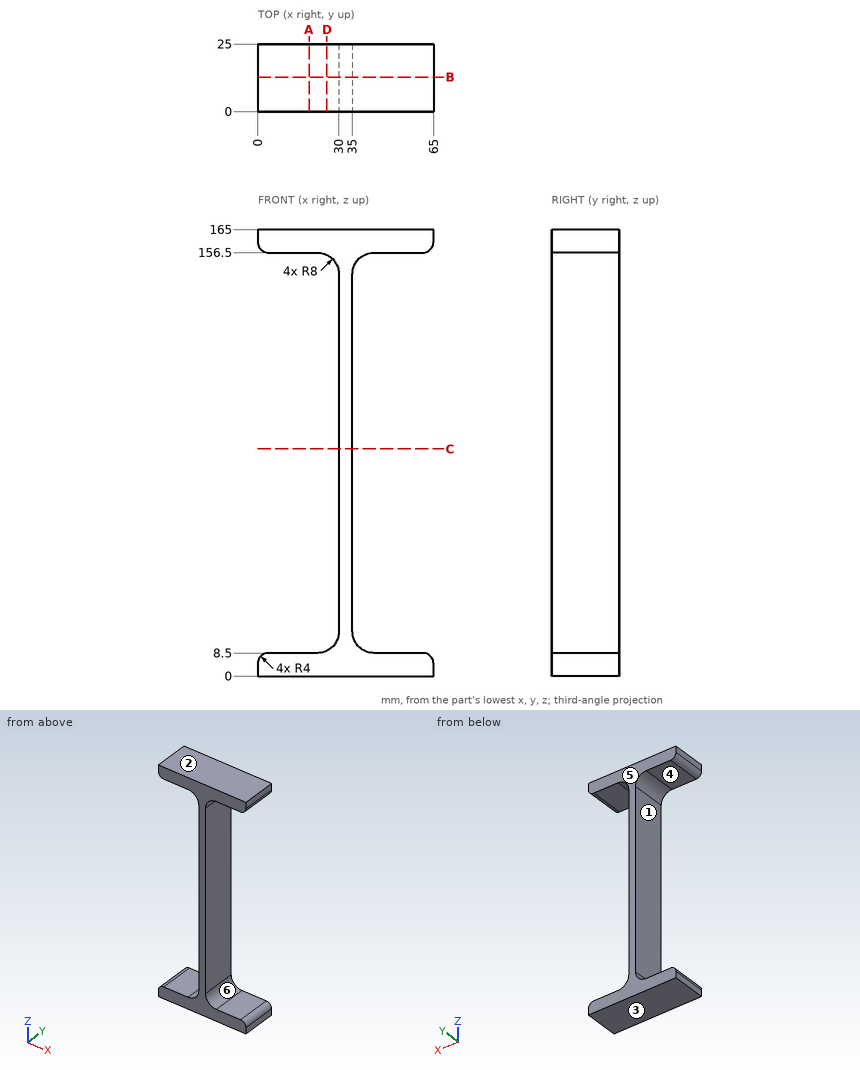
Source: three-view drawing plus pictorial views. Frame: mm from the lowest corner of the part. A direction names the side the tool comes from. Round coordinates to 2 decimals unless told otherwise and drop trailing zeros. Order: outer loops, then holes, each group sorted by start corner. A loop starts at its lowest first (then second) coordinate and runs counter-clockwise, first axis right, second up. Notation, with made-up numbers: (-14, 73) - (0, 73) arc R23 cw to (0, 91) - close; hole circle Ø5 at (44, 3). An arc over 180 degrees is marked (long way). Use a Markdown table: item, result.
1. Access query for the marked faces 4, 5 and 6. Directions: +Z, -Z, +X, -X, +Y, -Y. A direction counts if a zero-diameter tool reaches every point of the face in a straight line with its end or side. Return the directions, or none.
Evaluation:
| item | result |
|---|---|
| face 4 | -X, +Y, -Y |
| face 5 | +Z, -Z, +X, -X, +Y |
| face 6 | +X, +Y, -Y |
2. Section C-C on z = 84. Return the cut outline in (x, y), then the cut area to 3 significant figures.
Evaluation:
| item | result |
|---|---|
| outline | (30, 0) - (35, 0) - (35, 25) - (30, 25) - close |
| area | 125 mm^2 |
3. Section A-A on x = 19. Return the cut outline in (y, z), then the cut area to 3 significant figures.
Evaluation:
| item | result |
|---|---|
| outline | (0, 0) - (25, 0) - (25, 8.5) - (0, 8.5) - close; (0, 156.5) - (25, 156.5) - (25, 165) - (0, 165) - close |
| area | 425 mm^2 |
4. First-contact query: pin 1 (10 mm diameter, centred on y = 19.5, z = 105.5, fed in from -X). Flat tip, straight axial feed; report the tip coordinate or a pass-through.
Evaluation:
| item | result |
|---|---|
| pin 1 | x = 30 |
5. Section B-B on y = 12.75. Return the cut outline in (x, z).
Evaluation:
| item | result |
|---|---|
| outline | (0, 0) - (65, 0) - (65, 4.5) arc R4 ccw to (61, 8.5) - (43, 8.5) arc R8 cw to (35, 16.5) - (35, 148.5) arc R8 cw to (43, 156.5) - (61, 156.5) arc R4 ccw to (65, 160.5) - (65, 165) - (0, 165) - (0, 160.5) arc R4 ccw to (4, 156.5) - (22, 156.5) arc R8 cw to (30, 148.5) - (30, 16.5) arc R8 cw to (22, 8.5) - (4, 8.5) arc R4 ccw to (0, 4.5) - close |
6. Section D-D on x = 25.5. Return the cut outline in (y, z), then the cut area to 3 significant figures.
Evaluation:
| item | result |
|---|---|
| outline | (0, 0) - (25, 0) - (25, 9.31) - (0, 9.31) - close; (0, 155.69) - (25, 155.69) - (25, 165) - (0, 165) - close |
| area | 465 mm^2 |
7. Material intervals for probe 1 along Z at (x, y) = (12, 14.5); probe 2 along X at (y, z) = (1.75, 75); probe 3 along Z at (x, y) = (36.5, 13.5), sorted ascending.
Evaluation:
| item | result |
|---|---|
| probe 1 | 0 to 8.5, 156.5 to 165 |
| probe 2 | 30 to 35 |
| probe 3 | 0 to 11.84, 153.16 to 165 |
8. Mould query, pull axis Z, two halves, no side actions, for the marked faces 1, 2 and 3. Classes: +Z half, -Z half, draft (parallel to the pull), parting line (faces both ways), or undercut.
Evaluation:
| item | result |
|---|---|
| face 1 | undercut |
| face 2 | +Z half |
| face 3 | -Z half |
